```python
from build123d import *

# Parameters (mm, degrees)
SKETCH1_W                                  = 45.025374044
SKETCH1_H                                  = 45
BOSS_EXTRUDE1_DEPTH                        = 60
SKETCH2_R                                  = 21.1
CUT_EXTRUDE1_DEPTH                         = 8.8
SKETCH3_R                                  = 5.1
CUT_EXTRUDE2_DEPTH                         = 11.8
CHAMFER1_SIZE                              = 0.2
SKETCH4_R                                  = 14.5
CUT_EXTRUDE3_DEPTH                         = 79.305945349
SKETCH5_W                                  = 45.025374044
SKETCH5_H                                  = 45
CUT_EXTRUDE4_DEPTH                         = 14.8
SKETCH6_W                                  = 45.025374044
SKETCH6_H                                  = 23.350654293
CUT_EXTRUDE5_DEPTH                         = 24.8
FILLET3_R                                  = 5
FILLET4_R                                  = 5
FILLET7_R                                  = 5
FILLET8_R                                  = 5
BOSS_EXTRUDE3_START                        = 5
BOSS_EXTRUDE3_DEPTH                        = 5
SKETCH9_R                                  = 1.65
CUT_EXTRUDE6_DEPTH                         = 5
MIRROR2_AT_THE_SECOND_PLANE_COPY_1_SKETC_R = 1.65
MIRROR2_AT_THE_SECOND_PLANE_COPY_1_DEPTH   = 5


with BuildPart() as part:
    # Sketch1 → Boss-Extrude1 (new body)
    with BuildSketch(Plane(origin=(0, 0, 0), x_dir=(1, 0, 0), z_dir=(0, 1, 0))):
        Rectangle(SKETCH1_W, SKETCH1_H)
    extrude(amount=BOSS_EXTRUDE1_DEPTH)

    # Sketch2 → Cut-Extrude1 (cut)
    with BuildSketch(Plane(origin=(0, 60, 0), x_dir=(1, 0, 0), z_dir=(0, 1, 0))):
        with Locations(Location((0, 0, 0), (0, 0, 270))):
            Circle(SKETCH2_R)
    extrude(amount=-CUT_EXTRUDE1_DEPTH, mode=Mode.SUBTRACT)

    # Sketch3 → Cut-Extrude2 (cut)
    with BuildSketch(Plane(origin=(0, 51.2, 0), x_dir=(1, 0, 0), z_dir=(0, 1, 0))):
        with Locations(Location((0, 0, 0), (0, 0, 270))):
            Circle(SKETCH3_R)
    extrude(amount=-CUT_EXTRUDE2_DEPTH, mode=Mode.SUBTRACT)

    # Chamfer1
    chamfer1_edges = [part.edges().sort_by_distance(p)[0] for p in [
        (-22.512687022, 60, 0),
        (0, 51.2, -21.1),
        (0, 60, -21.1),
        (0, 60, 22.5),
        (22.512687022, 60, 0),
        (0, 60, -22.5),
    ]]
    chamfer(chamfer1_edges, length=CHAMFER1_SIZE)

    # Sketch4 → Cut-Extrude3 (cut, through all)
    with BuildSketch(Plane.XY.offset(22.5)):
        with Locations((0, 21.650654293)):
            Circle(SKETCH4_R)
    extrude(amount=-CUT_EXTRUDE3_DEPTH, mode=Mode.SUBTRACT)

    # Sketch5 → Cut-Extrude4 (cut)
    with BuildSketch(Plane.XZ):
        Rectangle(SKETCH5_W, SKETCH5_H)
    extrude(amount=-CUT_EXTRUDE4_DEPTH, mode=Mode.SUBTRACT)

    # Sketch6 → Cut-Extrude5 (cut)
    with BuildSketch(Plane.XY.offset(22.5)):
        with Locations((0, 26.475327146)):
            Rectangle(SKETCH6_W, SKETCH6_H)
    extrude(amount=-CUT_EXTRUDE5_DEPTH, mode=Mode.SUBTRACT)

    # Fillet3
    # the kernel refuses this fillet: 5 mm, written as the material it takes off along each edge
    with BuildSketch(Plane(origin=(22.512687022, 2.3, -22.5), x_dir=(0, 0, 1), z_dir=(0, 1, 0))) as fillet3_piece_1:
        with BuildLine():
            CenterArc((FILLET3_R, -FILLET3_R), FILLET3_R, 90, 90)
            Line((0, -FILLET3_R), (0, 0))
            Line((0, 0), (FILLET3_R, 0))
        make_face()
    extrude(amount=70, mode=Mode.SUBTRACT)

    # Fillet4
    # the kernel refuses this fillet: 5 mm, written as the material it takes off along each edge
    with BuildSketch(Plane(origin=(-22.512687022, 2.3, -22.5), x_dir=(0, 0, 1), z_dir=(0, 1, 0))) as fillet4_piece_1:
        with BuildLine():
            CenterArc((FILLET4_R, FILLET4_R), FILLET4_R, 180, 90)
            Line((0, FILLET4_R), (0, 0))
            Line((0, 0), (FILLET4_R, 0))
        make_face()
    extrude(amount=70, mode=Mode.SUBTRACT)

    # Fillet7
    # the kernel refuses this fillet: 5 mm, written as the material it takes off along each edge
    with BuildSketch(Plane(origin=(22.512687022, 25.650654293, 22.5), x_dir=(-1, 0, 0), z_dir=(0, 1, 0))) as fillet7_piece_1:
        with BuildLine():
            CenterArc((FILLET7_R, -FILLET7_R), FILLET7_R, 90, 90)
            Line((0, -FILLET7_R), (0, 0))
            Line((0, 0), (FILLET7_R, 0))
        make_face()
    extrude(amount=46.649345707, mode=Mode.SUBTRACT)

    # Fillet8
    # the kernel refuses this fillet: 5 mm, written as the material it takes off along each edge
    with BuildSketch(Plane(origin=(-22.512687022, 25.650654293, 22.5), x_dir=(1, 0, 0), z_dir=(0, 1, 0))) as fillet8_piece_1:
        with BuildLine():
            CenterArc((FILLET8_R, FILLET8_R), FILLET8_R, 180, 90)
            Line((0, FILLET8_R), (0, 0))
            Line((0, 0), (FILLET8_R, 0))
        make_face()
    extrude(amount=46.649345707, mode=Mode.SUBTRACT)

    # Sketch7 → Boss-Extrude3 (add)
    with BuildSketch(Plane.XY.offset(-2.3).offset(BOSS_EXTRUDE3_START)):
        with BuildLine():
            Line((-22.512687022, 14.8), (-12.779614069, 14.8))
            ThreePointArc((-12.779614069, 14.8), (-13.808706174, 17.22689641), (-14.381414349, 19.8))
            Line((-14.381414349, 19.8), (-22.512687022, 19.8))
            Line((-22.512687022, 19.8), (-22.512687022, 14.8))
        make_face()
    boss_extrude3 = extrude(amount=-BOSS_EXTRUDE3_DEPTH)

    # Mirror1: Boss-Extrude3 across plane
    add(boss_extrude3.mirror(Plane(origin=(0, 0, 0), x_dir=(0, 0, 1), z_dir=(1, 0, 0))))

    # Sketch9 → Cut-Extrude6 (cut)
    with BuildSketch(Plane(origin=(0, 60, 0), x_dir=(1, 0, 0), z_dir=(0, 1, 0))):
        with Locations(Location((-17.512687022, 17.5, 0), (0, 0, 270))):
            Circle(SKETCH9_R)
    cut_extrude6 = extrude(amount=-CUT_EXTRUDE6_DEPTH, mode=Mode.SUBTRACT)

    # Mirror2: Cut-Extrude6 across plane
    add(cut_extrude6.mirror(Plane(origin=(0, 0, 0), x_dir=(0, 0, 1), z_dir=(1, 0, 0))), mode=Mode.SUBTRACT)

    # Mirror2 at the second plane: Cut-Extrude6 across plane
    add(cut_extrude6.mirror(Plane.XY), mode=Mode.SUBTRACT)

    # Mirror2 at the second plane copy 1 sketc → Mirror2 at the second plane copy 1 (cut)
    with BuildSketch(Plane(origin=(0, 60, 0), x_dir=(-1, 0, 0), z_dir=(0, 1, 0))):
        with Locations(Location((-17.512687022, 17.5, 0), (0, 0, 270))):
            Circle(MIRROR2_AT_THE_SECOND_PLANE_COPY_1_SKETC_R)
    extrude(amount=-MIRROR2_AT_THE_SECOND_PLANE_COPY_1_DEPTH, mode=Mode.SUBTRACT)


solid = part.part
```
Verification items for the finished model (mm, model axes). A direction names the side the tool comes from. Round coordinates to 2 decimals unless told otherwise and drop trailing zeros. Order: outer loops, then holes, each group sorted by start corner. A loop starts at its lowest first (then second) coordinate and runs counter-clockwise, first axis right, second up.
1) Cross-section at C-C, the plane y = 25. Record the cut outline in (x, z), plus the area to 3 significant figures.
Geometry says:
outline: (-22.51, -17.5) arc R5 ccw to (-17.51, -22.5) - (-14.11, -22.5) - (-14.11, -2.3) - (-22.51, -2.3) - close; (14.11, -22.5) - (17.51, -22.5) arc R5 ccw to (22.51, -17.5) - (22.51, -2.3) - (14.11, -2.3) - close
area: 329 mm2
2) Draft check along Z on faces 6 (the cylindrical face through (-19.123, 57.535, -17.858)), 7 (the cylindrical face through (-21.087, 48.922, 20.996)), 8 (the flat face through (-8, 60, 20)). Enter one of: +Z half, -Z half, draft (parallel to the pull), parting line (faces both ways), or undercut.
Geometry says:
face 6: undercut
face 7: +Z half
face 8: draft
3) Cross-section at B-B, the plane x = 0. Record the cut outline in (y, z), plus the area to 3 significant figures.
Geometry says:
outline: (36.15, -22.5) - (59.8, -22.5) - (60, -22.3) - (60, -21.3) - (59.8, -21.1) - (51.4, -21.1) - (51.2, -20.9) - (51.2, -5.1) - (39.4, -5.1) - (39.4, 5.1) - (51.2, 5.1) - (51.2, 20.9) - (51.4, 21.1) - (59.8, 21.1) - (60, 21.3) - (60, 22.3) - (59.8, 22.5) - (38.15, 22.5) - (38.15, -2.3) - (36.15, -2.3) - close
area: 532 mm2
4) Depth check by flat-ended pin: pin 1 (5 mm diameter, centred on x = 14.5, z = 6.5, fed in from -Y); pin 2 (16.5 mm diameter, centred on x = 0, z = 0, fed in from -Y); pin 3 (14.5 mm diameter, centred on x = -5, y = 26.5, fed in from +Z); pin 4 (5.5 mm diameter, centred on x = -20.5, z = 1, fed in from +Y). Enter the tip coordinate at first touch or a pass-through.
Geometry says:
pin 1: stops at y = 38.15
pin 2: stops at y = 33.79
pin 3: passes through
pin 4: stops at y = 60
5) Tool access check on faces 1 (the flat face through (18, 17, 2.7)), 2 (the cylindrical face through (21.009, 48.922, 21.074)), 3 (the flat face through (0, 37, -2.3)), 4 (the cylindrical face through (1.532, 45.383, 4.864)), 5 (the cylindrical face through (-21.009, 37.084, -21.074)). Record the directions out of +Z, -Z, +X, -X, +Y, -Y that give a thin tool (end or side, any length) a straight path to the whole face; none if there is none.
Geometry says:
face 1: +Z, +X, -X, -Y
face 2: +Z, +X, +Y, -Y
face 3: +Z, +X, -X
face 4: +Y
face 5: -Z, -X, +Y, -Y
6) Material ranges on line 1 (X direction, y = 45, z = 0); line 2 (X direction, y = 58, z = 17); line 3 (X direction, y = 56.5, z = 0), recorded low to high.
Geometry says:
line 1: x = -22.51 to -5.1, 5.1 to 22.51
line 2: x = -22.51 to -19.09, -15.94 to -12.5, 12.5 to 15.94, 19.09 to 22.51
line 3: x = -22.51 to -21.1, 21.1 to 22.51
7) Cross-section at A-A, the plane z = 0. Record the cut outline in (x, y).
Geometry says:
outline: (-22.51, 14.8) - (-12.78, 14.8) arc R14.5 cw to (-14.38, 19.8) - (-22.51, 19.8) - close; (-22.51, 38.15) - (22.51, 38.15) - (22.51, 59.8) - (22.31, 60) - (21.3, 60) - (21.1, 59.8) - (21.1, 51.4) - (20.9, 51.2) - (5.1, 51.2) - (5.1, 39.4) - (-5.1, 39.4) - (-5.1, 51.2) - (-20.9, 51.2) - (-21.1, 51.4) - (-21.1, 59.8) - (-21.3, 60) - (-22.31, 60) - (-22.51, 59.8) - close; (12.78, 14.8) - (22.51, 14.8) - (22.51, 19.8) - (14.38, 19.8) arc R14.5 cw to start
